from build123d import *

# Parameters (mm, degrees)
SKETCH2_R           = 40
BOSS_EXTRUDE1_DEPTH = 920
SKETCH3_R           = 30
CUT_EXTRUDE1_DEPTH  = 900
CUT_EXTRUDE2_REACH  = 923.737
SKETCH4_R           = 22.5
BOSS_EXTRUDE2_START = 80
SKETCH5_R           = 40
BOSS_EXTRUDE2_DEPTH = 80
SKETCH6_W           = 40
SKETCH6_H           = 78
CUT_EXTRUDE3_DEPTH  = 5
SKETCH7_R           = 15
CUT_EXTRUDE4_DEPTH  = 924.91828643
FILLET2_R           = 5
FILLET3_R           = 2


with BuildPart() as part:
    # Sketch2 → Boss-Extrude1 (new body)
    with BuildSketch(Plane.XY):
        Circle(SKETCH2_R)
    extrude(amount=BOSS_EXTRUDE1_DEPTH)

    # Sketch3 → Cut-Extrude1 (cut)
    with BuildSketch(Plane(origin=(0, 0, 0), x_dir=(-1, 0, 0), z_dir=(0, 0, -1))):
        Circle(SKETCH3_R)
    extrude(amount=-CUT_EXTRUDE1_DEPTH, mode=Mode.SUBTRACT)

    # Sketch4 → Cut-Extrude2 (cut, up to next)
    with BuildSketch(Plane.XY.offset(920), mode=Mode.PRIVATE) as cut_extrude2_sk1:
        Circle(SKETCH4_R)
    cut_extrude2_tool1 = extrude(cut_extrude2_sk1.sketch, amount=-CUT_EXTRUDE2_REACH, mode=Mode.PRIVATE) & part.part
    add(cut_extrude2_tool1.solids().sort_by_distance((0, 0, 920))[0], mode=Mode.SUBTRACT)

    # Sketch5 → Boss-Extrude2 (add)
    with BuildSketch(Plane(origin=(0, 0, 0), x_dir=(-1, 0, 0), z_dir=(0, 0, -1)).offset(BOSS_EXTRUDE2_START)):
        Circle(SKETCH5_R)
    extrude(amount=-BOSS_EXTRUDE2_DEPTH)

    # Sketch6 → Cut-Extrude3 (cut)
    with BuildSketch(Plane(origin=(0, 40, 0), x_dir=(1, 0, 0), z_dir=(0, 1, 0))):
        with Locations((0, 41)):
            Rectangle(SKETCH6_W, SKETCH6_H)
    cut_extrude3 = extrude(amount=-CUT_EXTRUDE3_DEPTH, mode=Mode.SUBTRACT)

    # Mirror1: Cut-Extrude3 across plane
    add(cut_extrude3.mirror(Plane.ZX), mode=Mode.SUBTRACT)

    # Sketch7 → Cut-Extrude4 (cut, through all)
    with BuildSketch(Plane(origin=(0, 35, 0), x_dir=(1, 0, 0), z_dir=(0, 1, 0))):
        with Locations(Location((0, 45, 0), (0, 0, 270))):
            Circle(SKETCH7_R)
    extrude(amount=-CUT_EXTRUDE4_DEPTH, mode=Mode.SUBTRACT)

    # Fillet2
    fillet2_edges = [part.edges().sort_by_distance(p)[0] for p in [
        (40, 0, -80),
        (0, 35, -80),
        (-34.457195687, 20.315060063, -80),
        (0, -35, -80),
        (-40, 0, 920),
    ]]
    fillet(fillet2_edges, radius=FILLET2_R - 0.0001)  # a hair under: the kernel refuses the full size

    # Fillet3
    fillet3_edges = [part.edges().sort_by_distance(p)[0] for p in [
        (0, -35, -60),
        (0, 35, -60),
    ]]
    fillet(fillet3_edges, radius=FILLET3_R)


solid = part.part
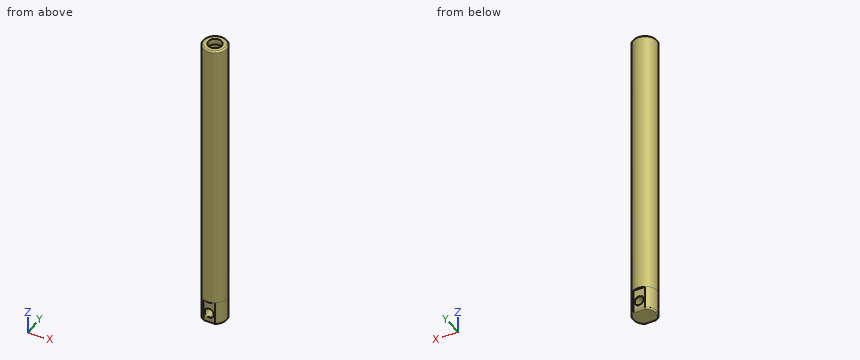
Model file for the job. Use its own axes, mm. Round coordinates to 2 decimals unless told otherwise and drop trailing zeros. Loops run counter-clockwise (first coordinate to the right, second up) from the corner with the lowest first, then second, coordinate; pieces in that order, holes last. Notation, with made-up numbers: (64.25, 7) - (104.25, 7) arc R23 ccw to (104.25, 15) - close; hole circle Ø1 at (41.25, 13). An arc over 180 degrees is marked (long way). Write each question's results on one line, items separated by ' | '.
(1) Saw through at B-B, the plane x = 0. List the corners of the cut face in (y, z), then the cut area to 3 significant figures.
Answer below:
outline: (-40, -2) - (-35, -2) - (-35, -28) arc R2 ccw to (-33, -30) - (33, -30) arc R2 ccw to (35, -28) - (35, -2) - (40, -2) - (40, 915) arc R5 ccw to (35, 920) - (22.5, 920) - (22.5, 900) - (30, 900) - (30, 0) - (-30, 0) - (-30, 900) - (-22.5, 900) - (-22.5, 920) - (-35, 920) arc R5 ccw to (-40, 915) - close; (-35, -75) arc R5 ccw to (-30, -80) - (30, -80) arc R5 ccw to (35, -75) - (35, -62) arc R2 ccw to (33, -60) - (-33, -60) arc R2 ccw to (-35, -62) - close | area: 22,200 mm^2
(2) Saw through at A-A, the plane z = -45. List the corners of the cut face in (x, y), then the cut area to 3 significant figures.
Answer below:
outline: (-19.36, -35) - (-17, -35) arc R2 ccw to (-15, -33) - (-15, 33) arc R2 ccw to (-17, 35) - (-19.36, 35) arc R40 ccw to start; (15, -33) arc R2 ccw to (17, -35) - (19.36, -35) arc R40 ccw to (19.36, 35) - (17, 35) arc R2 ccw to (15, 33) - close | area: 2,660 mm^2
(3) Wall check: L1, parallel to Z at x = -25.5, y = -3; L2, parallel to Y at x = -24, z = 659; L3, parallel to X at y = 25, z = 220.5. Give the ranges that are in metal, low to high.
Answer below:
L1: z = -80 to 0, 900 to 920 | L2: y = -32 to -18, 18 to 32 | L3: x = -31.22 to -16.58, 16.58 to 31.22
(4) Saw through at C-C, the plane z = 725.5. List the corners of the cut face in (x, y), then the cut area to 3 significant figures.
Answer below:
outline: circle Ø80 at (0, 0); hole circle Ø60 at (0, 0) | area: 2,200 mm^2
(5) Pin check, flat tips, straight feed: pin 1 (8 mm diameter, centred on y = -11, z = 761, fed in from -X); pin 2 (10 mm diameter, centred on x = -20.5, z = 469.5, fed in from -Y); pin 3 (5 mm diameter, centred on y = -5.5, z = 421.5, fed in from -X). Stop position of each tip, or through.
Answer below:
pin 1: stops at x = -39.38 | pin 2: stops at y = -36.87 | pin 3: stops at x = -39.89
